Read the model definition and answer for the solid it produces. Units are mm, in the model's axes. A direction names the side the tool comes from. Round coordinates to 2 decimals unless told otherwise and drop trailing zeros. Order: outer loops, then holes, each group sorted by start corner. A loop starts at its lowest first (then second) coordinate and runs counter-clockwise, first axis right, second up. Notation, with made-up numbers: (26, 59) -> (38, 59) arc R11 ccw to (38, 69) -> close; hole circle Ø2 at (22.25, 65.5). An arc over 180 degrees is marked (long way). Answer as a JSON object with one key per item and string values. Group by question number.
Item 1: Section C-C, the plane x = 42.5 is taken. Write down the section's boundary in (y, z).
Item 2: Section D-D, the plane z = 14 is taken. Write down the section's boundary in (x, y).
Item 3: Consider probe 1 along X at (y, z) = (4.5, 10.75); probe 2 along Z at (x, y) = (47.5, 14); probe 3 along X at (y, z) = (1.5, 27). Determine where each line is inside the solid, lowest interval first. Write a range as from..to.
Item 4: The mould has two halves that part along X. Classify faces 1 (the flat face through (52.324, -10, 14)), 2 (the flat face through (-46, -33, 28.448)), 3 (the flat face through (-34.798, -29, 25)): pulls with the +X half, pulls with the -X half, needs draft (parallel to the pull), parting line crosses it, or undercut.
Item 5: Section A-A, the plane y = 4 is taken. Write down the section's boundary in (x, z), plus the area to 3 significant figures.
Item 6: Given P1, Ø1.9, axis at y = 22.5, z = 4, coming from the +X side; P2, Ø2, axis at x = -33.5, z = 8.5, coming from the -Y side; P3, Ø8.5, axis at x = 3.5, z = 14.5, coming from the -Y side; P4, Ø4, axis at x = 41.5, y = 5, coming from the +Z side, each flat-ended and moving along its own axis, determine where each tip first touches the part or whether it passes through.
Item 7: Section B-B, the plane z = 2.75 is taken. Write down the section's boundary in (x, y), plus the area to 3 significant figures.
Item 8: For faces 4 (the flat face through (-38, 41, 15.748)), 5 (the flat face through (41, -28.956, 3)), 6 (the flat face through (-37.84, -34.34, 14.02)), 7 (the flat face through (43.688, 2, 14)), determine the directions among +Z, -Z, +X, -X, +Y, -Y from which every point of the face is accessible in a straight line to the end or side of a thin tool.
from build123d import *

# Parameters (mm, degrees)
F0_W      = 28.575
F0_H      = 88.9
F0_W_2    = 47.498
F1_DEPTH  = 28.448
F2_DEPTH  = 25.4
F3_W      = 28.575
F3_H      = 73.406
F4_DEPTH  = 6.35
F5_W      = 28.575
F5_H      = 6.35
F6_DEPTH  = 6.35
F7_DEPTH  = 12.7
F8_W      = 47.498
F8_H      = 25.4
F9_DEPTH  = 28.449
F11_DEPTH = 28.449


with BuildPart() as f1:
    # F0 (on Top) → F1 (new body)
    with BuildSketch(Plane.XY):
        with Locations((-38.0365, 0)):
            Rectangle(F0_W, F0_H)
        with BuildLine():
            ThreePointArc((-43.688, 14.224), (-38.1, 19.812), (-32.512, 14.224))
            Line((-32.512, 14.224), (-32.512, -9.652))
            ThreePointArc((-32.512, -9.652), (-38.1, -15.24), (-43.688, -9.652))
            Line((-43.688, -9.652), (-43.688, 14.224))
        make_face(mode=Mode.SUBTRACT)
        Rectangle(F0_W_2, F0_H)
        with Locations((38.0365, 0)):
            Rectangle(F0_W, F0_H)
        with BuildLine():
            ThreePointArc((32.512, 14.224), (38.1, 19.812), (43.688, 14.224))
            Line((43.688, 14.224), (43.688, -9.652))
            ThreePointArc((43.688, -9.652), (38.1, -15.24), (32.512, -9.652))
            Line((32.512, -9.652), (32.512, 14.224))
        make_face(mode=Mode.SUBTRACT)
    extrude(amount=F1_DEPTH)

    # F0 (on Top) → F2 (join)
    with BuildSketch(Plane.XY):
        with Locations((-38.0365, 0)):
            Rectangle(F0_W, F0_H)
        with BuildLine():
            ThreePointArc((-43.688, 14.224), (-38.1, 19.812), (-32.512, 14.224))
            Line((-32.512, 14.224), (-32.512, -9.652))
            ThreePointArc((-32.512, -9.652), (-38.1, -15.24), (-43.688, -9.652))
            Line((-43.688, -9.652), (-43.688, 14.224))
        make_face(mode=Mode.SUBTRACT)
        Rectangle(F0_W_2, F0_H)
        with Locations((38.0365, 0)):
            Rectangle(F0_W, F0_H)
        with BuildLine():
            ThreePointArc((32.512, 14.224), (38.1, 19.812), (43.688, 14.224))
            Line((43.688, 14.224), (43.688, -9.652))
            ThreePointArc((43.688, -9.652), (38.1, -15.24), (32.512, -9.652))
            Line((32.512, -9.652), (32.512, 14.224))
        make_face(mode=Mode.SUBTRACT)
    extrude(amount=F2_DEPTH)

    # F3 (on face) → F4 (cut)
    with BuildSketch(Plane(origin=(0, 0, 0), x_dir=(1, 0, 0), z_dir=(0, 0, -1))):
        with Locations((38.0365, -7.747)):
            Rectangle(F3_W, F3_H)
        with BuildLine():
            ThreePointArc((43.688, -14.224), (38.1, -19.812), (32.512, -14.224))
            Line((32.512, -14.224), (32.512, 9.652))
            ThreePointArc((32.512, 9.652), (38.1, 15.24), (43.688, 9.652))
            Line((43.688, 9.652), (43.688, -14.224))
        make_face(mode=Mode.SUBTRACT)
        with Locations((-38.0365, -7.747)):
            Rectangle(F3_W, F3_H)
        with BuildLine():
            Line((-32.512, 9.652), (-32.512, -14.224))
            ThreePointArc((-32.512, -14.224), (-38.1, -19.812), (-43.688, -14.224))
            Line((-43.688, -14.224), (-43.688, 9.652))
            ThreePointArc((-43.688, 9.652), (-38.1, 15.24), (-32.512, 9.652))
        make_face(mode=Mode.SUBTRACT)
    extrude(amount=-F4_DEPTH, mode=Mode.SUBTRACT)

    # F5 (on face) → F6 (cut)
    with BuildSketch(Plane.XY.offset(28.448)):
        with Locations((38.0365, 41.275)):
            Rectangle(F5_W, F5_H)
        Polygon((-23.749, 38.1), (-52.324, 38.1), (-52.324, -25.146), (-34.798, -25.146), (-34.798, -44.45), (-23.749, -44.45), align=None)
        with BuildLine():
            Line((-43.688, -9.652), (-43.688, 14.224))
            ThreePointArc((-43.688, 14.224), (-38.1, 19.812), (-32.512, 14.224))
            Line((-32.512, 14.224), (-32.512, -9.652))
            ThreePointArc((-32.512, -9.652), (-38.1, -15.24), (-43.688, -9.652))
        make_face(mode=Mode.SUBTRACT)
        with Locations((-38.0365, 41.275)):
            Rectangle(F5_W, F5_H)
        Polygon((52.324, 38.1), (23.749, 38.1), (23.749, -44.45), (34.798, -44.45), (34.798, -25.146), (52.324, -25.146), align=None)
        with BuildLine():
            ThreePointArc((43.688, -9.652), (38.1, -15.24), (32.512, -9.652))
            Line((32.512, -9.652), (32.512, 14.224))
            ThreePointArc((32.512, 14.224), (38.1, 19.812), (43.688, 14.224))
            Line((43.688, 14.224), (43.688, -9.652))
        make_face(mode=Mode.SUBTRACT)
    extrude(amount=-F6_DEPTH, mode=Mode.SUBTRACT)

    # F5 (on face) → F7 (cut)
    with BuildSketch(Plane.XY.offset(28.448)):
        with Locations((-38.0365, 41.275)):
            Rectangle(F5_W, F5_H)
        with Locations((38.0365, 41.275)):
            Rectangle(F5_W, F5_H)
    extrude(amount=-F7_DEPTH, mode=Mode.SUBTRACT)

    # F8 (on face) → F9 (cut, through all)
    with BuildSketch(Plane.XY.offset(28.448)):
        with Locations((0, -31.75)):
            Rectangle(F8_W, F8_H)
    extrude(amount=-F9_DEPTH, mode=Mode.SUBTRACT)

    # F10 (on face) → F11 (cut, through all)
    with BuildSketch(Plane.XY):
        Polygon((-23.749, -24.506965), (-52.324, -44.45), (-23.749, -44.45), align=None)
        Polygon((23.749, -44.45), (52.668778, -44.45), (23.749, -24.506965), align=None)
    extrude(amount=F11_DEPTH, mode=Mode.SUBTRACT)


solid = f1.part
Values found:
{
 "1": {"outline": "(-37.44, 0) -> (-28.96, 0) -> (-28.96, 6.35) -> (-13.1, 6.35) -> (-13.1, 22.1) -> (-25.15, 22.1) -> (-25.15, 28.45) -> (-37.44, 28.45) -> close; (17.67, 6.35) -> (44.45, 6.35) -> (44.45, 15.75) -> (38.1, 15.75) -> (38.1, 22.1) -> (17.67, 22.1) -> close"},
 "2": {"outline": "(-52.32, -44.45) -> (-23.75, -24.51) -> (-23.75, -19.05) -> (23.75, -19.05) -> (23.75, -24.51) -> (52.32, -44.21) -> (52.32, 44.45) -> (-52.32, 44.45) -> close; hole (-43.69, -9.65) arc R5.59 ccw to (-32.51, -9.65) -> (-32.51, 14.22) arc R5.59 ccw to (-43.69, 14.22) -> close; hole (32.51, -9.65) arc R5.59 ccw to (43.69, -9.65) -> (43.69, 14.22) arc R5.59 ccw to (32.51, 14.22) -> close"},
 "3": {"probe 1": "-52.32..-43.69, -32.51..32.51, 43.69..52.32", "probe 2": "6.35..22.1", "probe 3": "-23.75..23.75"},
 "4": {"face 1": "pulls with the +X half", "face 2": "needs draft", "face 3": "undercut"},
 "5": {"outline": "(-52.32, 6.35) -> (-43.69, 6.35) -> (-43.69, 22.1) -> (-52.32, 22.1) -> close; (-32.51, 6.35) -> (-23.75, 6.35) -> (-23.75, 0) -> (23.75, 0) -> (23.75, 6.35) -> (32.51, 6.35) -> (32.51, 22.1) -> (23.75, 22.1) -> (23.75, 28.45) -> (-23.75, 28.45) -> (-23.75, 22.1) -> (-32.51, 22.1) -> close; (43.69, 6.35) -> (52.32, 6.35) -> (52.32, 22.1) -> (43.69, 22.1) -> close", "area": "1,900 mm2"},
 "6": {"P1": "x = 23.75", "P2": "y = -32.01", "P3": "y = -19.05", "P4": "through"},
 "7": {"outline": "(-52.32, -44.45) -> (-30.12, -28.96) -> (-52.32, -28.96) -> close; (-23.75, -19.05) -> (23.75, -19.05) -> (23.75, 44.45) -> (-23.75, 44.45) -> close; (30.2, -28.96) -> (52.32, -44.21) -> (52.32, -28.96) -> close", "area": "3,360 mm2"},
 "8": {"face 4": "+Z, -X, +Y", "face 5": "-Z, +X, -X, +Y", "face 6": "+Z, -Z, -Y", "face 7": "+Z, -Z"}
}
